Study the drawing (mm; zero at the part's minimum x, y, z) and answer. A direction names the side the tool comes from. Give positions to 0.01 mm unless a question says otherwise; leave off trailing zeros. Write each loop counter-clockwise with the first axis right and the second up, starting at its lowest first coordinate (ties: lowest second). Pieces come first, ordered by that corner, then holes. Notation, with made-up numbers: (77.5, -9) - (136.5, -9) arc R18 ccw to (136.5, -2) - close; hole circle Ø9 at (54, -3.75). An arc over 180 degrees is marked (long way). Write each question's results on one line, items separated by ' | '. Start each with the question number.
Q1. For a pull along X with two mould halves and no side action, classify the marked faces 3, 4 and 5 as pulls with the +X half, pulls with the -X half, needs draft (parallel to the pull), parting line crosses it, or undercut.
Q2. For the marked faces 1 and 2, determine the directions among +Z, -Z, +X, -X, +Y, -Y from which every point of the face is accessible in a straight line to the end or side of a thin tool.
Q3. Section D-D (y = 9.5) is taken. Determine the outline of the cut face in (x, z).
Q4. Flat-ended cylindrical pins translate along their axes: pin 1 Ø2.5 at (x, y) = (87, 20) entering from +Z; pin 2 Ø3 at (x, z) = (23.5, 1) entering from +Y. Find the tip coordinate at first contact, or state that the pin passes through.
Q5. Section B-B (y = 17) is taken. Determine the outline of the cut face in (x, z).
Q6. Find the intervals of material crossed by probe 1 along Y at (x, z) = (3, 3.5); probe 2 along Y at (x, z) = (5, 7.75); probe 3 along Z at (x, y) = (79.5, 19.5), in increasing order.
Q7. Section C-C (y = 28) is taken. Determine the outline of the cut face in (x, z) (1 decimal).
Q8. Section A-A (x = 3) is taken. Determine the outline of the cut face in (y, z).
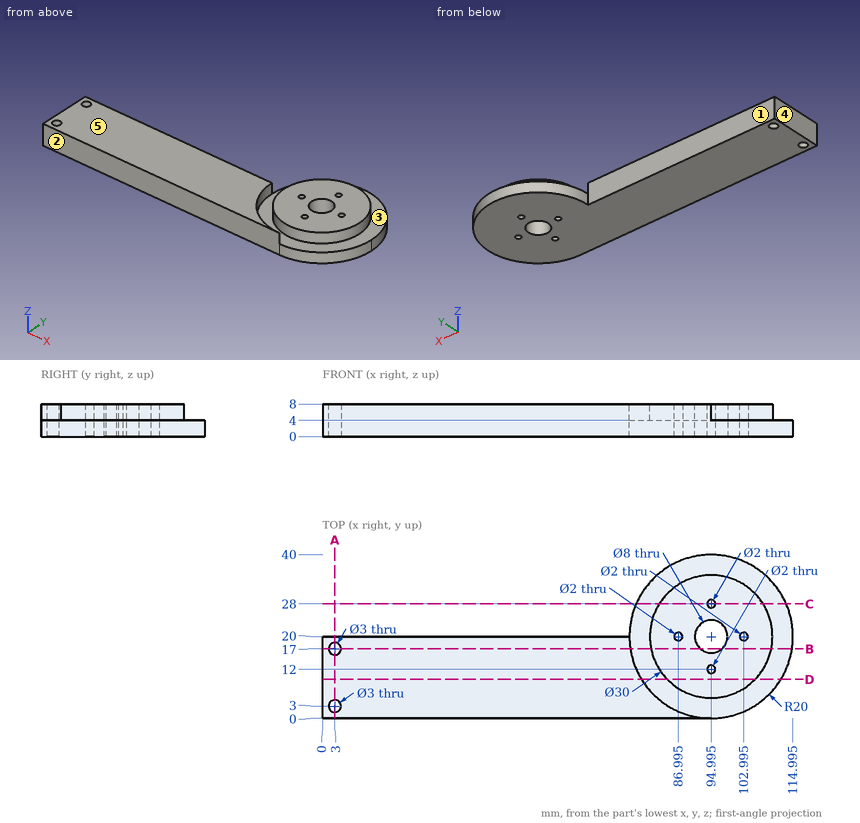
Answers below:
1) face 3: undercut | face 4: pulls with the -X half | face 5: needs draft
2) face 1: +Z, -Z, -X, +Y | face 2: +Z, -Z, +X, -X, -Y
3) outline: (0, 0) - (112.02, 0) - (112.02, 4) - (105.71, 4) - (105.71, 8) - (84.28, 8) - (84.28, 4) - (77.97, 4) - (77.97, 8) - (0, 8) - close
4) pin 1: stops at z = 8 | pin 2: stops at y = 20
5) outline: (0, 0) - (1.5, 0) - (1.5, 8) - (0, 8) - close; (4.5, 0) - (92.35, 0) - (92.35, 8) - (80.3, 8) - (80.3, 4) - (75.22, 4) - (75.22, 8) - (4.5, 8) - close; (97.64, 0) - (114.77, 0) - (114.77, 4) - (109.69, 4) - (109.69, 8) - (97.64, 8) - close
6) probe 1: y = 0 to 1.5, 4.5 to 15.5, 18.5 to 20 | probe 2: y = 0 to 20 | probe 3: z = 0 to 4
7) outline: (76.7, 0) - (94, 0) - (94, 8) - (82.3, 8) - (82.3, 4) - (76.7, 4) - close; (96, 0) - (113.3, 0) - (113.3, 4) - (107.7, 4) - (107.7, 8) - (96, 8) - close
8) outline: (0, 0) - (1.5, 0) - (1.5, 8) - (0, 8) - close; (4.5, 0) - (15.5, 0) - (15.5, 8) - (4.5, 8) - close; (18.5, 0) - (20, 0) - (20, 8) - (18.5, 8) - close
